Geometry check sheet. Reference: the model listing, model coordinates, mm. A direction names the side the tool comes from. Round coordinates to 2 decimals unless told otherwise and drop trailing zeros. Order: outer loops, then holes, each group sorted by start corner. A loop starts at its lowest first (then second) coordinate and runs counter-clockwise, first axis right, second up. Notation, with made-up numbers: (16.5, -14.75) - (56.5, -14.75) arc R19 cw to (56.5, -1.75) - close; hole circle Ø8 at (-12, 70.5). An arc over 180 degrees is marked (long way). Write each question's results on one line, items separated by ' | '.
```python
from build123d import *

# Parameters (mm, degrees)
SKETCH1_W           = 2.8
SKETCH1_H           = 2.8
BOSS_EXTRUDE1_DEPTH = 17
BOSS_EXTRUDE2_START = 6.5
SKETCH1_3_W         = 4.55
SKETCH1_3_H         = 2.8
BOSS_EXTRUDE2_DEPTH = 2


with BuildPart() as part:
    # Sketch1 → Boss-Extrude1 (new body)
    with BuildSketch(Plane.XY):
        with Locations((2.375, 1.5)):
            Rectangle(SKETCH1_W, SKETCH1_H)
    extrude(amount=BOSS_EXTRUDE1_DEPTH)

    # Sketch1<3> → Boss-Extrude2 (add)
    with BuildSketch(Plane.XY.offset(BOSS_EXTRUDE2_START)):
        with Locations((2.375, 1.5)):
            Rectangle(SKETCH1_3_W, SKETCH1_3_H)
    extrude(amount=BOSS_EXTRUDE2_DEPTH)


solid = part.part
```
(1) Access from +Z, -Z, +X, -X, +Y, -Y to the whole of each face (thin tool, end or side, straight path). Record for faces 1 (the face through (3.775, 1, 3)), 2 (the face through (4, 2, 8.5)), 3 (the face through (0.5, 1.5, 6.5)), 4 (the face through (0.5, 1.5, 8.5)).
Answers follow:
face 1: -Z, +X, +Y, -Y | face 2: +Z, +X, +Y, -Y | face 3: -Z, -X, +Y, -Y | face 4: +Z, -X, +Y, -Y
(2) Material ranges on line 1 (X direction, y = 1.3, z = 15) (3 decimals); line 2 (Z direction, x = 0.7, y = 2.6), recorded low to high.
Answers follow:
line 1: 0.975 to 3.775 | line 2: 6.5 to 8.5
(3) Section check A-A (y = 1.9). Record the cut outline in (x, z) (3 decimals), then the cut area to 3 significant figures.
Answers follow:
outline: (0.1, 6.5) - (0.975, 6.5) - (0.975, 0) - (3.775, 0) - (3.775, 6.5) - (4.65, 6.5) - (4.65, 8.5) - (3.775, 8.5) - (3.775, 17) - (0.975, 17) - (0.975, 8.5) - (0.1, 8.5) - close | area: 51.1 mm²
(4) Depth check by flat-ended pin: pin 1 Ø0.8 at (y, z) = (1, 13.5) entering from -X (3 decimals). Enter the tip coordinate at first touch or a pass-through.
Answers follow:
pin 1: x = 0.975
(5) Section check B-B (z = 14.25). Record the cut outline in (x, y) (3 decimals).
Answers follow:
outline: (0.975, 0.1) - (3.775, 0.1) - (3.775, 2.9) - (0.975, 2.9) - close
